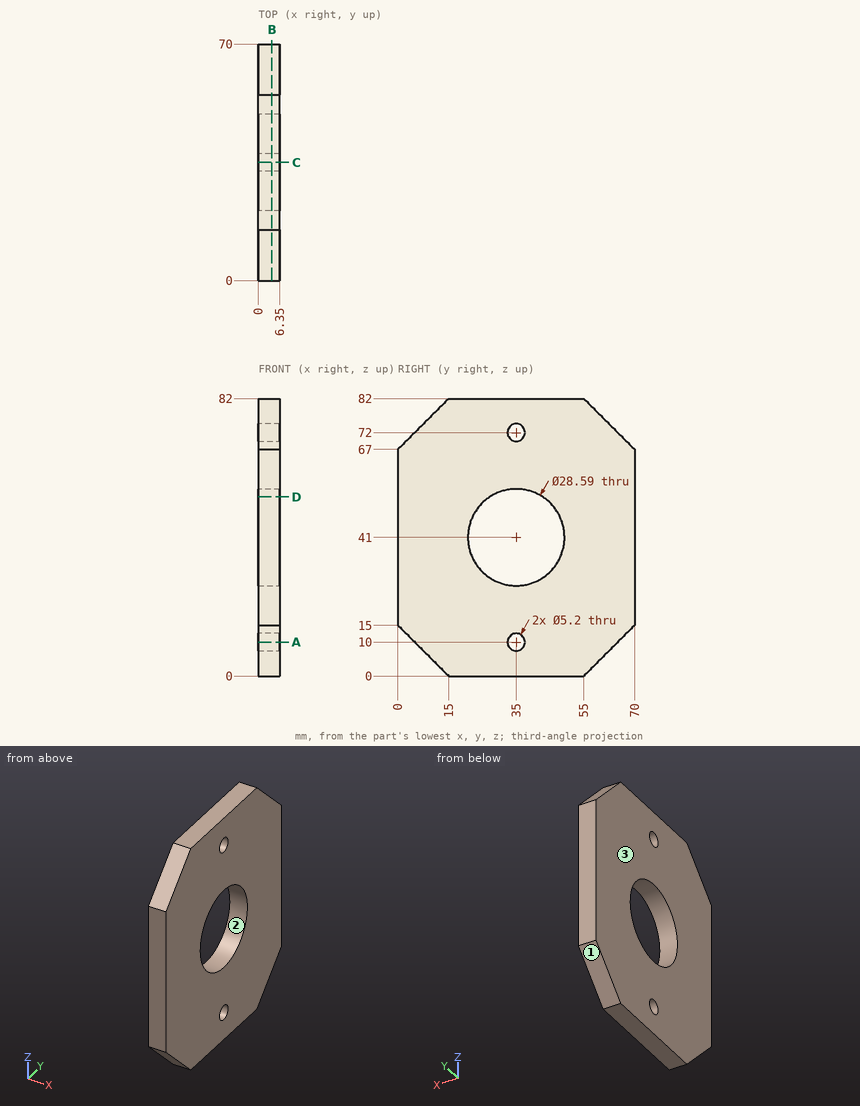
Design review of the part shown in the three views and the two pictorial views. Dimensions are in mm from the part's minimum x, y and z. Round coordinates to 2 decimals unless told otherwise and drop trailing zeros. Loops run counter-clockwise (first coordinate to the right, second up) from the corner with the lowest first, then second, coordinate; pieces in that order, holes last. Notation, with made-up numbers: (85, 35) - (138, 35) arc R8 cw to (138, 48) - close; hole circle Ø9 at (64.5, 16). An arc over 180 degrees is marked (long way). Write each question's results on one line, items separated by ' | '. Start each with the question number.
Q1. Insertion check: P1, Ø10, axis at y = 23.5, z = 41.5, coming from the -X side; P2, Ø2, axis at x = 3, z = 13.5, coming from the -Y side. Each pin has a flat end and moves straight along its axis. Give the tip position at first contact, or say it passes through.
Q2. Take a section at B-B on x = 4. Give the boundary of the cut face in (y, z) (3 decimals), plus the area to 3 significant figures.
Q3. Draft analysis for pull direction Y (two halves, no side actions). For the marked faces 1, 2 and 3, state which applies: pulls with the +Y half, pulls with the -Y half, needs draft (parallel to the pull), parting line crosses it, or undercut.
Q4. Take a section at C-C on y = 35. Give the boundary of the cut face in (x, z) (3 decimals), plus the area to 3 significant figures.
Q5. Take a section at A-A on z = 10. Give the boundary of the cut face in (x, y), plus the area to 3 significant figures.
Q6. Wall thickness on line 1 along Y through (x, z) = (5.5, 41) (3 decimals); line 2 along Y through (x, z) = (3, 72); line 3 along Y through (x, z) = (3.5, 5.5): over which ranges is each line inside the solid? List them lowest first. Write a range as [from, to].
Q7. Take a section at D-D on z = 53. Give the boundary of the cut face in (x, y), plus the area to 3 significant figures.
Data:
1) P1: stops at x = 0 | P2: stops at y = 0.5
2) outline: (0, 15) - (15, 0) - (55, 0) - (70, 15) - (70, 67) - (55, 82) - (15, 82) - (0, 67) - close; hole circle Ø28.59 at (35, 41); hole circle Ø5.2 at (35, 10); hole circle Ø5.2 at (35, 72) | area: 4,610 mm²
3) face 1: pulls with the +Y half | face 2: undercut | face 3: needs draft
4) outline: (0, 0) - (6.35, 0) - (6.35, 7.4) - (0, 7.4) - close; (0, 12.6) - (6.35, 12.6) - (6.35, 26.705) - (0, 26.705) - close; (0, 55.295) - (6.35, 55.295) - (6.35, 69.4) - (0, 69.4) - close; (0, 74.6) - (6.35, 74.6) - (6.35, 82) - (0, 82) - close | area: 273 mm²
5) outline: (0, 5) - (6.35, 5) - (6.35, 32.4) - (0, 32.4) - close; (0, 37.6) - (6.35, 37.6) - (6.35, 65) - (0, 65) - close | area: 348 mm²
6) line 1: y = [0, 20.705], [49.295, 70] | line 2: y = [5, 32.4], [37.6, 65] | line 3: y = [9.5, 60.5]
7) outline: (0, 0) - (6.35, 0) - (6.35, 27.23) - (0, 27.23) - close; (0, 42.77) - (6.35, 42.77) - (6.35, 70) - (0, 70) - close | area: 346 mm²
